Source: CAD feature listing. Evaluate the final solid. Frame: model axes, mm. A direction names the side the tool comes from. Round coordinates to 2 decimals unless told otherwise and drop trailing zeros. Order: outer loops, then holes, each group sorted by start corner. A loop starts at its lowest first (then second) coordinate and runs counter-clockwise, first axis right, second up.
Autodesk Inventor part; units mm, degrees
ref_plane "YZ Plane" through (0, 0, 0) normal (1, 0, 0) x (0, 1, 0)
ref_plane "XZ Plane" through (0, 0, 0) normal (0, 1, 0) x (-1, 0, 0)
ref_plane "XY Plane" through (0, 0, 0) normal (0, 0, 1) x (1, 0, 0)
sketch "Sketch1" plane through (0, 0, 0) normal (0, 1, 0) x (-1, 0, 0)
  circle A0 centre (0, 0) radius 7
  dimension "d0" = 14
extrude "Extrusion1" add sketch "Sketch1" along normal blind 158
sketch "Sketch2" plane through (0, 158, 0) normal (0, 1, 0) x (1, 0, 0)
  circle A0 centre (0, 0) radius 3.75
  line L0 (-5.25, -1.5) -> (-2.25, -1.5)
  line L1 (-2.25, -1.5) -> (-2.25, 1.5)
  line L2 (-2.25, 1.5) -> (-5.25, 1.5)
  line L3 (-5.25, 1.5) -> (-5.25, -1.5)
  line L4 (-5.25, -1.5) -> (-2.25, 1.5) construction
  line L5 (-2.25, -1.5) -> (-5.25, 1.5) construction
  line L6 (-1.5, 2.25) -> (1.5, 2.25)
  line L7 (1.5, 2.25) -> (1.5, 5.25)
  line L8 (1.5, 5.25) -> (-1.5, 5.25)
  line L9 (-1.5, 5.25) -> (-1.5, 2.25)
  line L10 (-1.5, 2.25) -> (1.5, 5.25) construction
  line L11 (1.5, 2.25) -> (-1.5, 5.25) construction
  line L12 (2.25, 1.5) -> (5.25, 1.5)
  line L13 (5.25, 1.5) -> (5.25, -1.5)
  line L14 (5.25, -1.5) -> (2.25, -1.5)
  line L15 (2.25, -1.5) -> (2.25, 1.5)
  line L16 (2.25, 1.5) -> (5.25, -1.5) construction
  line L17 (5.25, 1.5) -> (2.25, -1.5) construction
  line L18 (-1.5, -5.25) -> (1.5, -5.25)
  line L19 (1.5, -5.25) -> (1.5, -2.25)
  line L20 (1.5, -2.25) -> (-1.5, -2.25)
  line L21 (-1.5, -2.25) -> (-1.5, -5.25)
  line L22 (-1.5, -5.25) -> (1.5, -2.25) construction
  line L23 (1.5, -5.25) -> (-1.5, -2.25) construction
  point P0 (-3.75, 0)
  point P1 (0, 3.75)
  point P2 (3.75, 0)
  point P3 (0, -3.75)
  point P4 (-3.4369, -1.5)
  point P5 (-1.5, -3.4369)
  point P6 (1.5, -3.4369)
  point P7 (3.4369, -1.5)
  point P8 (3.4369, 1.5)
  point P9 (1.5, 3.4369)
  point P10 (-1.5, 3.4369)
  point P11 (-3.4369, 1.5)
  dimension "d58" = 7.5
  dimension "d59" = 3
  dimension "d60" = 3
  dimension "d61" = 3
  dimension "d62" = 3
  dimension "d63" = 3
  dimension "d64" = 3
  dimension "d65" = 3
  dimension "d66" = 3
extrude "Extrusion2" cut sketch "Sketch2" against normal through all
sketch "Sketch3" plane through (0, 158, 0) normal (0, 1, 0) x (1, 0, 0)
  circle A0 centre (0, 0) radius 9
  line L0 (-0.258, -9) -> (-0.258, -9)
  line L1 (-0.258, -11) -> (-0.258, -11)
  line L2 (-0.5, -9.5) -> (0.5, -9.5)
  line L3 (0.5, -9.5) -> (0.5, -8.5)
  line L4 (0.5, -8.5) -> (-0.5, -8.5)
  line L5 (-0.5, -8.5) -> (-0.5, -9.5)
  line L6 (-0.5, -9.5) -> (0.5, -8.5) construction
  line L7 (0.5, -9.5) -> (-0.5, -8.5) construction
  line L8 (-0.5, 8.5) -> (0.5, 8.5)
  line L9 (0.5, 8.5) -> (0.5, 9.5)
  line L10 (0.5, 9.5) -> (-0.5, 9.5)
  line L11 (-0.5, 9.5) -> (-0.5, 8.5)
  line L12 (-0.5, 8.5) -> (0.5, 9.5) construction
  line L13 (0.5, 8.5) -> (-0.5, 9.5) construction
  point P0 (0.492, 8.9865)
  point P1 (-0.258, -8.9963)
  point P2 (0, -9)
  point P3 (0, 9)
  point P4 (0.5, -8.9861)
  point P5 (-0.5, -8.9861)
  point P6 (-0.5, 8.9861)
  point P7 (0.5, 8.9861)
  dimension "d15" = 18
  dimension "d19" = 9
  dimension "d36" = 1
  dimension "d37" = 1
  dimension "d38" = 1
  dimension "d39" = 1
extrude "Extrusion3" cut sketch "Sketch3" against normal blind 8
sketch "Sketch5" plane through (0, 0, 0) normal (0, -1, 0) x (1, 0, 0)
  line L0 (-1.25, 3.25) -> (-1.25, 1.25)
  line L1 (-1.25, 1.25) -> (-3.25, 1.25)
  line L2 (3.25, 1.25) -> (1.25, 1.25)
  line L3 (1.25, 1.25) -> (1.25, 3.25)
  line L4 (1.25, -3.25) -> (1.25, -1.25)
  line L5 (1.25, -1.25) -> (3.25, -1.25)
  line L6 (-3.25, -1.25) -> (-1.25, -1.25)
  line L7 (-1.25, -1.25) -> (-1.25, -3.25)
  circle A0 centre (0, 0) radius 3.75
  line L8 (-3.4369, -1.5) -> (-5.25, -1.5)
  line L9 (-2.25, 1.5) -> (-5.25, 1.5)
  line L10 (-5.25, 1.5) -> (-5.25, -1.5)
  line L11 (-5.25, -1.5) -> (-2.25, -1.5)
  line L12 (-2.25, -1.5) -> (-2.25, 1.5)
  line L13 (-2.25, 1.5) -> (-5.25, -1.5) construction
  line L14 (-5.25, 1.5) -> (-2.25, -1.5) construction
  line L15 (-1.5, -5.25) -> (-1.5, -3.4369)
  line L16 (1.5, -2.25) -> (-1.5, -2.25)
  line L17 (-1.5, -2.25) -> (-1.5, -5.25)
  line L18 (-1.5, -5.25) -> (1.5, -5.25)
  line L19 (1.5, -5.25) -> (1.5, -2.25)
  line L20 (1.5, -2.25) -> (-1.5, -5.25) construction
  line L21 (-1.5, -2.25) -> (1.5, -5.25) construction
  line L22 (1.5, 2.25) -> (-1.5, 2.25)
  line L23 (-1.5, 2.25) -> (-1.5, 5.25)
  line L24 (-1.5, 5.25) -> (1.5, 5.25)
  line L25 (1.5, 5.25) -> (1.5, 2.25)
  line L26 (1.5, 2.25) -> (-1.5, 5.25) construction
  line L27 (-1.5, 2.25) -> (1.5, 5.25) construction
  line L28 (5.25, 1.5) -> (5.25, -1.5)
  line L29 (2.25, 1.5) -> (5.25, 1.5)
  line L30 (5.25, 1.5) -> (5.25, -1.5)
  line L31 (5.25, -1.5) -> (2.25, -1.5)
  line L32 (2.25, -1.5) -> (2.25, 1.5)
  line L33 (2.25, 1.5) -> (5.25, -1.5) construction
  line L34 (5.25, 1.5) -> (2.25, -1.5) construction
  point P0 (-3.25, 3.25)
  point P1 (3.25, -3.25)
  point P2 (-3.75, 0)
  point P3 (0, -3.75)
  point P4 (0, 3.75)
  point P5 (3.75, 0)
  point P6 (3.4369, -1.5)
  point P7 (3.4369, 1.5)
  point P8 (-1.5, 3.4369)
  point P9 (1.5, 3.4369)
  point P10 (-3.4369, 1.5)
  point P11 (1.5, -3.4369)
  dimension "d54" = 360
extrude "Extrusion5" add sketch "Sketch5" against normal blind 30 contours L23 L24 L25 A0 | A0 L8 L10 L9 | L29 L28 L31 A0 | A0 L19 L18 L15
sketch "Sketch6" plane through (0, 150, 0) normal (0, 1, 0) x (1, 0, 0)
  circle A0 centre (0, 0) radius 7
  line L0 (0, 0) -> (7, 0) construction
  circle A1 centre (-4.9497, 4.9497) radius 1
  circle A2 centre (-4.9497, -4.9497) radius 1
  circle A3 centre (4.9497, -4.9497) radius 1
  circle A4 centre (4.9497, 4.9497) radius 1
  dimension "d69" = 2
  dimension "d70" = 4.9497
  dimension "d71" = 4.9497
  dimension "d74" = 360
extrude "Extrusion6" cut sketch "Sketch6" against normal blind 2 contours A4 A0 | A0 A4 | A3 A0 | A0 A3 | A1 A0 | A0 A1 | A2 A0 | A0 A2
properties part number "Upper Arm" material "PLA Plastic"
1. Section A-A on x = 0. Return loops of the section in (y, z).
2. Section C-C on y = 91. Return loops of the section in (x, z).
3. Section D-D on y = 23. Return loops of the section in (x, z).
4. Line query: line 1 along X through (y, z) = (40, 0); line 2 along Y through (x, z) = (-1.25, 4.75). Output: solid intervals per line, ascending.
5. Section B-B on z = 0. Return loops of the section in (x, y), plus the area to 3 significant figures.
6. Pull-direction query (Z, two-part tool) for faces 1 (the face through (-6.466, 73.95, 2.681)), 2 (the face through (5.25, 91, 0)), 3 (the face through (-3.368, 59.383, -1.65)), 4 (the face through (3, 150, 3)); classes: released by +Z, released by -Z, zero draft, split by the parting line, or undercut.
7. First-contact query: pin 1 (0.8 mm diameter, centred on x = 4.5, z = -5, fed in from +Y); pin 2 (2 mm diameter, centred on x = -4.5, y = 82.5, fed in from -Z); pin 3 (2 mm diameter, centred on y = 101.5, z = 5, fed in from +X). Flat tips, straight axial feed; report the tip coordinate or a pass-through.
8. Access query for faces 5 (the face through (-3, 0, -3)), 6 (the face through (0, 91, -5.25)). Directions: +Z, -Z, +X, -X, +Y, -Y. A direction counts if a zero-diameter tool reaches every point of the face in a straight line with its end or side. Return the directions, or none.
Result:
1. outline: (0, -7) - (150, -7) - (150, -5.25) - (30, -5.25) - (30, -3.75) - (0, -3.75) - close; (0, 3.75) - (30, 3.75) - (30, 5.25) - (150, 5.25) - (150, 7) - (0, 7) - close
2. outline: circle Ø14 at (0, 0); hole (-5.25, -1.5) - (-3.44, -1.5) arc R3.75 ccw to (-1.5, -3.44) - (-1.5, -5.25) - (1.5, -5.25) - (1.5, -3.44) arc R3.75 ccw to (3.44, -1.5) - (5.25, -1.5) - (5.25, 1.5) - (3.44, 1.5) arc R3.75 ccw to (1.5, 3.44) - (1.5, 5.25) - (-1.5, 5.25) - (-1.5, 3.44) arc R3.75 ccw to (-3.44, 1.5) - (-5.25, 1.5) - close
3. outline: circle Ø14 at (0, 0); hole circle Ø7.5 at (0, 0)
4. line 1: x = -7 to -5.25, 5.25 to 7
4. line 2: y = 0 to 30
5. outline: (-7, 0) - (-3.75, 0) - (-3.75, 30) - (-5.25, 30) - (-5.25, 150) - (-7, 150) - close; (3.75, 0) - (7, 0) - (7, 150) - (5.25, 150) - (5.25, 30) - (3.75, 30) - close
5. area: 615 mm2
6. face 1: split by the parting line
6. face 2: undercut
6. face 3: undercut
6. face 4: zero draft
7. pin 1: stops at y = 148
7. pin 2: stops at z = -6.06
7. pin 3: stops at x = 5.74
8. face 5: +Z, -Z, +X, -X, -Y
8. face 6: +Y
